Source: CAD feature listing. Evaluate the final solid. Frame: model axes, mm. Give positions to 0.01 mm unless a question says otherwise; leave off trailing zeros. Loops run counter-clockwise (first coordinate to the right, second up) from the corner with the lowest first, then second, coordinate; pieces in that order, holes last. Notation, with made-up numbers: M -29,68 L 12,68 A31 ccw 12,97 Z; hole C 67.5,-34 d2. An arc over 180 degrees is marked long. Answer in a Markdown table with one row per item.
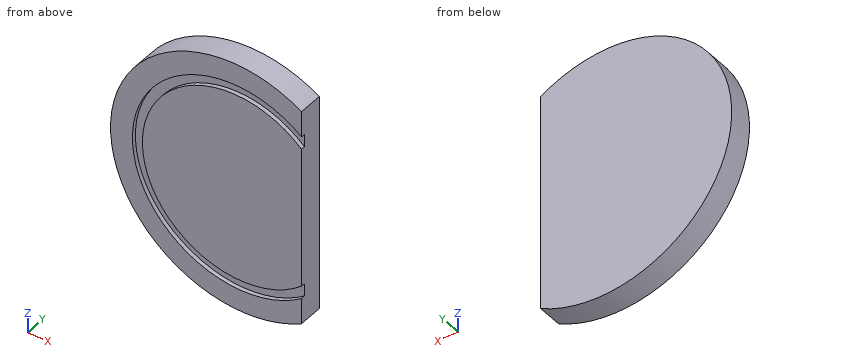
```python
from build123d import *

# Parameters (mm, degrees)
BOSS_EXTRUDE1_DEPTH = 19.05
SKETCH2_R           = 84.1375
SKETCH2_R_2         = 76.2
CUT_EXTRUDE1_DEPTH  = 3.175


with BuildPart() as part:
    # Sketch1 → Boss-Extrude1 (new body)
    with BuildSketch(Plane(origin=(0, 0, 0), x_dir=(1, 0, 0), z_dir=(0, 1, 0))):
        with BuildLine():
            Line((50.8, -87.988181024), (50.8, 87.988181024))
            ThreePointArc((50.8, 87.988181024), (-101.6, 0), (50.8, -87.988181024))
        make_face()
    extrude(amount=BOSS_EXTRUDE1_DEPTH)

    # Sketch2 → Cut-Extrude1 (cut)
    with BuildSketch(Plane.XZ):
        Circle(SKETCH2_R)
        Circle(SKETCH2_R_2, mode=Mode.SUBTRACT)
    extrude(amount=-CUT_EXTRUDE1_DEPTH, mode=Mode.SUBTRACT)


solid = part.part
```
1) Section C-C, the plane y = 7. Return loops of the section in (x, z), then the cut area to 3 significant figures.
Reply:
| item | result |
|---|---|
| outline | M 50.8,-87.99 L 50.8,87.99 A101.6 ccw long Z |
| area | 26,100 mm² |
2) Section B-B, the plane z = 70. Return loops of the section in (x, y) (3 decimals), then the cut area to 3 significant figures.
Reply:
| item | result |
|---|---|
| outline | M -73.638,0 L -46.681,0 L -46.681,3.175 L -30.107,3.175 L -30.107,0 L 30.107,0 L 30.107,3.175 L 46.681,3.175 L 46.681,0 L 50.8,0 L 50.8,19.05 L -73.638,19.05 Z |
| area | 2,270 mm² |
3) Section A-A, the plane x = -81.5. Return loops of the section in (y, z) (3 decimals), then the cut area to 3 significant figures.
Reply:
| item | result |
|---|---|
| outline | M 0,-60.666 L 19.05,-60.666 L 19.05,60.666 L 0,60.666 L 0,20.901 L 3.175,20.901 L 3.175,-20.901 L 0,-20.901 Z |
| area | 2,180 mm² |
4) Material intervals for L1, parallel to Z at x = 0, y = 0.7; L2, parallel to Z at x = 43, y = 1.25; L3, parallel to X at y = 5, z = 57, sorted ascending.
Reply:
| item | result |
|---|---|
| L1 | z = -101.6 to -84.14, -76.2 to 76.2, 84.14 to 101.6 |
| L2 | z = -92.05 to -72.32, -62.91 to 62.91, 72.32 to 92.05 |
| L3 | x = -84.1 to 50.8 |
5) Section D-D, the plane x = -9. Return loops of the section in (y, z) (3 decimals).
Reply:
| item | result |
|---|---|
| outline | M 0,-101.201 L 19.05,-101.201 L 19.05,101.201 L 0,101.201 L 0,83.655 L 3.175,83.655 L 3.175,75.667 L 0,75.667 L 0,-75.667 L 3.175,-75.667 L 3.175,-83.655 L 0,-83.655 Z |
6) Pin query (flat end, axial travel): pin 1 Ø2 at (y, z) = (3.5, -22) entering from -X; pin 2 Ø1 at (x, y) = (-55.5, 6) entering from -Z; pin 3 Ø1 at (x, y) = (15.5, 5.5) entering from -Z. Return the tip coordinate at first contact, or that it passes through.
Reply:
| item | result |
|---|---|
| pin 1 | stops at x = -99.41 |
| pin 2 | stops at z = -85.43 |
| pin 3 | stops at z = -100.49 |
